Autodesk Inventor part; units mm, degrees
ref_plane "YZ Plane" through (0, 0, 0) normal (1, 0, 0) x (0, 1, 0)
ref_plane "XZ Plane" through (0, 0, 0) normal (0, 1, 0) x (-1, 0, 0)
ref_plane "XY Plane" through (0, 0, 0) normal (0, 0, 1) x (1, 0, 0)
sketch "Esboço1" plane through (0, 0, 0) normal (0, 0, 1) x (1, 0, 0)
  line L0 (0, 0) -> (50, 0)
  line L1 (50, 0) -> (50, 65)
  line L2 (50, 65) -> (0, 65)
  line L3 (0, 65) -> (0, 0)
  circle A0 centre (25, 45) radius 6
  dimension "d0" = 50
  dimension "d1" = 65
  dimension "d2" = 12
  dimension "d8" = 45
  dimension "d14" = 25
extrude "Extrusão1" add sketch "Esboço1" along normal blind 5
sketch "Esboço2" plane through (0, 0, 5) normal (0, 0, 1) x (1, 0, 0)
  line L0 (50, 0) -> (50, 65)
  line L1 (0, 0) -> (50, 0)
  line L2 (50, 0) -> (50, 5)
  line L3 (50, 5) -> (0, 5)
  line L4 (0, 5) -> (0, 0)
  dimension "d5" = 5
extrude "Extrusão2" add sketch "Esboço2" along normal blind 70
sketch "Esboço3" plane through (0, 5, 5) normal (0, 1, 0) x (1, 0, 0)
  circle A0 centre (25, -45) radius 6
  line L0 (50, -70) -> (0, -70)
  line L1 (50, 0) -> (50, -70)
  point P0 (0, 5)
  dimension "d9" = 12
  dimension "d10" = 25
  dimension "d11" = 25
extrude "Extrusão3" cut sketch "Esboço3" against normal blind 40
properties part number "Teste Suporte"
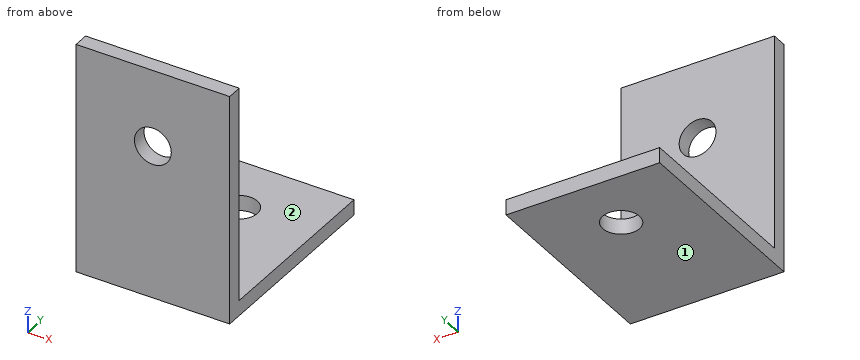
Part model, mm, in its own coordinate system. Face numbers are marked on the shaded views. A direction names the side the tool comes from. Round coordinates to 2 decimals unless told otherwise and drop trailing zeros. Loops run counter-clockwise (first coordinate to the right, second up) from the corner with the lowest first, then second, coordinate; pieces in that order, holes last. Notation, with made-up numbers: (15.25, 35.5) -> (24.25, 35.5) arc R33 cw to (24.25, 63.5) -> close; hole circle Ø3 at (72.5, -10.5). An arc over 180 degrees is marked (long way). Use CSV: the item, a comma, the result in double quotes. Start each with the question number.
1) Which spindle directions (+Z, -Z, +X, -X, +Y, -Y) get a long thin tool onto all of the face, cutting with end or side? Do the marked faces 1 and 2. Say none if no direction does.
2) Cut at D-D, the plane x = 41.5. Write the cut outline in (y, z).
3) Drop flat-ended pins along their axis: P1, Ø3, axis at x = 24, z = 10.5, coming from the +Y side; P2, Ø4, axis at x = 12.5, y = 41.5, coming from the +Z side. Give the stop position or say it passes through.
4) Wall check: L1, parallel to Z at x = 25, y = 3.45; L2, parallel to X at y = 2.45, z = 50; L3, parallel to Y at x = 25, z = 3.95. Give the ranges that are in metal, low to high. Write a range as [from, to].
5) Cut at A-A, the plane x = 25. Write the cut outline in (y, z), plus the area to 3 significant figures.
6) Cut at B-B, the plane z = 50. Write the cut outline in (x, y).
Determined:
1,face 1,"-Z, +X, -X, +Y, -Y"
1,face 2,"+Z, +X, -X, +Y"
2,outline,"(0, 0) -> (65, 0) -> (65, 5) -> (5, 5) -> (5, 75) -> (0, 75) -> close"
3,P1,"stops at y = 5"
3,P2,"stops at z = 5"
4,L1,"z = [0, 44], [56, 75]"
4,L2,"x = [0, 19], [31, 50]"
4,L3,"y = [0, 39], [51, 65]"
5,outline,"(0, 0) -> (39, 0) -> (39, 5) -> (5, 5) -> (5, 44) -> (0, 44) -> close; (0, 56) -> (5, 56) -> (5, 75) -> (0, 75) -> close; (51, 0) -> (65, 0) -> (65, 5) -> (51, 5) -> close"
5,area,"555 mm2"
6,outline,"(0, 0) -> (19, 0) -> (19, 5) -> (0, 5) -> close; (31, 0) -> (50, 0) -> (50, 5) -> (31, 5) -> close"
